Build history of the part. All positions in model axes, mm. Face numbers are marked on the shaded views. A direction names the side the tool comes from. Round coordinates to 2 decimals unless told otherwise and drop trailing zeros. Order: outer loops, then holes, each group sorted by start corner. A loop starts at its lowest first (then second) coordinate and runs counter-clockwise, first axis right, second up. Notation, with made-up numbers: M 44.5,-14.75 L 82.5,-14.75 A24 cw 82.5,1.25 Z; hole C 6,50 d9. An arc over 180 degrees is marked long. One line per item, written item: value. Start each with the question number.
Item 1: Two-plate mould, pull along Y, no slides. Class the marked faces 6, 7 and 8: +Y half, -Y half, draft (parallel to the pull), parting line (faces both ways), or undercut.
Item 2: Band-saw the part on A-A, the plane z = 42. Write the cut outline in (x, y), then the cut area to 3 significant figures.
Item 3: Tool access for the marked faces 1, 2, 3, 4 and 5: list every direction of +Z, -Z, +X, -X, +Y, -Y with a clear straight run to the whole face (end or side of a thin tool).
Item 4: Band-saw the part on B-B, the plane y = -15.5. Give the number of separate pieces and of enclosed holes in the cut face, then the cut area to 3 significant figures.
Item 5: Band-saw the part on D-D, the plane z = 11.5. Write the cut outline in (x, y), then the cut area to 3 significant figures.
Item 6: Band-saw the part on C-C, the plane x = 57.5. Write the cut outline in (y, z).
Item 7: Pin check, flat tips, straight feed: pin 1 (4 mm diameter, centred on x = 75, z = 27.5, fed in from -Y); pin 2 (1.5 mm diameter, centred on x = 86, y = -29.5, fed in from +Z); pin 3 (4.5 mm diameter, centred on x = 109, y = -39, fed in from +Z); pin 4 (4 mm diameter, centred on x = 54, y = -14.5, fed in from +Z). Stop position of each tip, or through.
Item 8: Probe L1, parallel to X at y = -12, z = 17; L2, parallel to X at y = -10, z = 13.5; L3, parallel to Z at x = 83, y = -23. List the from-to ranges inside material, lowest first.
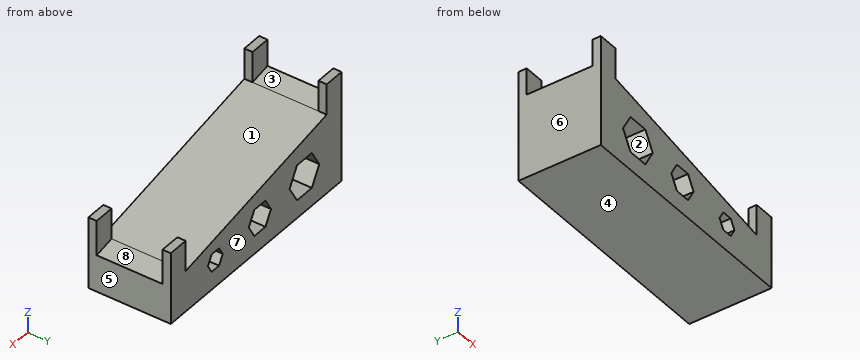
```python
from build123d import *

# Parameters (mm, degrees)
PAD_DEPTH    = 40
SKETCH001_W  = 142.064534
SKETCH001_H  = 32
POCKET_DEPTH = 35.197263


with BuildPart() as part:
    # Sketch → Pad (new body)
    with BuildSketch(Plane.XZ):
        Polygon((0, 0), (0, 53.896675), (10, 53.896675), (10, 38.896675), (105, 20), (105, 35), (115, 35), (115, 0), align=None)
        Polygon((30, 8.839746), (35, 17.5), (30, 26.160254), (20, 26.160254), (15, 17.5), (20, 8.839746), align=None, mode=Mode.SUBTRACT)
        Polygon((58.75, 8.839746), (62.5, 15.334936), (58.75, 21.830127), (51.25, 21.830127), (47.5, 15.334936), (51.25, 8.839746), align=None, mode=Mode.SUBTRACT)
        Polygon((87.5, 8.839746), (90, 13.169873), (87.5, 17.5), (82.5, 17.5), (80, 13.169873), (82.5, 8.839746), align=None, mode=Mode.SUBTRACT)
    extrude(amount=PAD_DEPTH)

    # Sketch001 (on Face4 of Pad) → Pocket (cut, through all)
    with BuildSketch(Plane(origin=(7.823159, 0, 39.329676), x_dir=(-0.980785, 0, 0.19509), z_dir=(0.19509, 0, 0.980785))):
        with Locations((-56.611011, 20)):
            Rectangle(SKETCH001_W, SKETCH001_H)
    extrude(amount=POCKET_DEPTH, mode=Mode.SUBTRACT)


solid = part.part
```
Output:
1. face 6: draft
1. face 7: +Y half
1. face 8: undercut
2. outline: M 0,-40 L 10,-40 L 10,-36 L 0,-36 Z; M 0,-4 L 10,-4 L 10,0 L 0,0 Z
2. area: 80.0 mm²
3. face 1: +Z, +Y, -Y
3. face 2: +Y, -Y
3. face 3: +Z, +X
3. face 4: -Z, +X, -X, +Y, -Y
3. face 5: +Z, -Z, +X, +Y, -Y
4. separate pieces: 1
4. enclosed holes: 3
4. area: 2,920 mm²
5. outline: M 0,-40 L 18.46,-40 L 18.46,0 L 0,0 Z; M 31.54,-40 L 49.71,-40 L 49.71,0 L 31.54,0 Z; M 60.29,-40 L 80.96,-40 L 80.96,0 L 60.29,0 Z; M 89.04,-40 L 115,-40 L 115,0 L 89.04,0 Z
5. area: 3,330 mm²
6. outline: M -40,0 L 0,0 L 0,8.84 L -40,8.84 Z; M -40,21.83 L 0,21.83 L 0,29.45 L -40,29.45 Z
7. pin 1: stops at y = -40
7. pin 2: stops at z = 23.93
7. pin 3: stops at z = 35
7. pin 4: stops at z = 30.54
8. L1: x = 0 to 15.29, 34.71 to 48.46, 61.54 to 82.21, 87.79 to 115
8. L2: x = 0 to 17.31, 32.69 to 48.56, 61.44 to 80.19, 89.81 to 115
8. L3: z = 0 to 8.84, 17.5 to 24.38
